```python
from build123d import *

# Parameters (mm, degrees)
SKETCH1_W                = 50
SKETCH1_H                = 50
BOSS_EXTRUDE1_DEPTH      = 50
CUT_EXTRUDE2_DEPTH       = 87.602540378
CUT_EXTRUDE3_DEPTH       = 40
CHAMFER1_SIZE            = 4
CHAMFER3_SIZE            = 1.5
BOSS_EXTRUDE2_DEPTH      = 7
BOSS_EXTRUDE2_DEPTH_BACK = 10
SKETCH5_W                = 1
SKETCH5_H                = 7
SKETCH6_W                = 1.8
SKETCH6_H                = 1.8
CUT_EXTRUDE4_DEPTH       = 7


with BuildPart() as part:
    # Sketch1 → Boss-Extrude1 (new body)
    with BuildSketch(Plane.XY):
        with Locations((25, 25)):
            Rectangle(SKETCH1_W, SKETCH1_H)
    extrude(amount=BOSS_EXTRUDE1_DEPTH)

    # Sketch3 → Cut-Extrude2 (cut, through all)
    with BuildSketch(Plane.XZ):
        Polygon((29.556349186, 39), (36, 45.443650814), (36, 54.556349186), (29.556349186, 61), (20.443650814, 61), (14, 54.556349186), (14, 45.443650814), (20.443650814, 39), align=None)
    extrude(amount=-CUT_EXTRUDE2_DEPTH, mode=Mode.SUBTRACT)

    # Sketch4 → Cut-Extrude3 (cut)
    with BuildSketch(Plane.XY.offset(50)):
        Polygon((33.69848481, 46), (16.30151519, 46), (4, 33.69848481), (4, 16.30151519), (16.30151519, 4), (33.69848481, 4), (46, 16.30151519), (46, 33.69848481), align=None)
    extrude(amount=-CUT_EXTRUDE3_DEPTH, mode=Mode.SUBTRACT)

    # Chamfer1
    chamfer1_edges = [part.edges().sort_by_distance(p)[0] for p in [
        (10.150757595, 10.150757595, 10),
        (10.150757595, 39.849242405, 10),
        (39.849242405, 39.849242405, 10),
        (39.849242405, 10.150757595, 10),
        (25, 4, 10),
        (25, 46, 10),
        (46, 25, 10),
        (4, 25, 10),
    ]]
    chamfer(chamfer1_edges, length=CHAMFER1_SIZE)

    # Chamfer3
    chamfer3_edges = [part.edges().sort_by_distance(p)[0] for p in [
        (50, 25, 50),
        (43, 50, 50),
        (43, 0, 50),
        (7, 50, 50),
        (36, 46.849242405, 50),
        (14, 3.150757595, 50),
        (14, 50, 47.721825407),
        (36, 50, 47.721825407),
        (36, 0, 47.721825407),
        (14, 0, 47.721825407),
        (17.221825407, 0, 42.221825407),
        (32.778174593, 0, 42.221825407),
        (17.221825407, 50, 42.221825407),
        (32.778174593, 50, 42.221825407),
        (0, 25, 50),
        (25, 50, 0),
        (50, 25, 0),
        (36, 3.150757595, 50),
        (14, 46.849242405, 50),
        (25, 0, 0),
        (9, 11.30151519, 50),
        (9, 38.69848481, 50),
        (4, 25, 50),
        (41, 38.69848481, 50),
        (0, 25, 0),
        (41, 11.30151519, 50),
        (46, 25, 50),
        (7, 0, 50),
        (0, 50, 25),
        (50, 50, 25),
        (50, 0, 25),
        (0, 0, 25),
    ]]
    chamfer(chamfer3_edges, length=CHAMFER3_SIZE)

    # Sketch5 → Boss-Extrude2 (add, two sides: drawn at the far end of the back side and taken through both)
    with BuildSketch(Plane.XY.offset(50).offset(-BOSS_EXTRUDE2_DEPTH_BACK)):
        with Locations((49.5, 25)):
            Rectangle(SKETCH5_W, SKETCH5_H)
    extrude(amount=BOSS_EXTRUDE2_DEPTH + BOSS_EXTRUDE2_DEPTH_BACK)

    # Sketch6 → Cut-Extrude4 (cut)
    with BuildSketch(Plane(origin=(50, 0, 0), x_dir=(0, 0, -1), z_dir=(1, 0, 0))):
        with Locations((-53.6, 25)):
            Rectangle(SKETCH6_W, SKETCH6_H)
    extrude(amount=-CUT_EXTRUDE4_DEPTH, mode=Mode.SUBTRACT)


solid = part.part
```
The model under review builds one solid part; all positions refer to its coordinate system, in mm. A direction names the side the tool comes from. Round coordinates to 2 decimals unless told otherwise and drop trailing zeros. Order: outer loops, then holes, each group sorted by start corner. A loop starts at its lowest first (then second) coordinate and runs counter-clockwise, first axis right, second up. Notation, with made-up numbers: (-9, -17.75) -> (16, -17.75) arc R24 ccw to (16, 16.25) -> close; hole circle Ø10 at (-7, -22). An arc over 180 degrees is marked (long way). One line per item, written item: value. Start each with the question number.
Q1. Take a section at D-D (y = 31). Write out the cut boundary in (x, z).
Q2. Take a section at A-A (y = 25). Write out the cut boundary in (x, z), and give its area (3 significant figures).
Q3. Take a section at C-C (x = 21.5). Write out the cut boundary in (y, z).
Q4. Mouldability with a two-part tool opening along X and no side actions: class faces 6 (the face through (10.2, 39.9, 31.5)), 7 (the face through (0.8, 0.7, 24.7)), 8 (the face through (42.9, 0.8, 49.3)) as released by +X, released by -X, zero draft, split by the parting line, or undercut.
Q5. Wall thickness on line 1 (X direction, y = 22, z = 17); line 2 (Z direction, x = 47, y = 4): over which ranges is each line inside the solid? List them lowest first.
Q6. Take a section at B-B (z = 26). Write out the cut boundary in (x, y), and give its area (3 significant figures).
Q7. Clearance check with flat-ended pins moving along their axes: pin 1 Ø0.5 at (x, z) = (49.5, 52) entering from -Y; pin 2 Ø0.5 at (x, z) = (49.5, 54) entering from +Y; pin 3 Ø5.5 at (x, y) = (45.5, 14) entering from +Z. State where each tip first meets the part, or that it passes through.
Q8. Machinability: for faces 1 (the face through (25, 46, 29)), 2 (the face through (6.9, 0.7, 49.2)), 3 (the face through (13, 1, 49)), 4 (the face through (36.7, 46.1, 49.2)), 5 (the face through (25, 25, 0)), which of the approach directions +Z, -Z, +X, -X, +Y, -Y give a long, thin tool a straight path to every point of the face, cutting with its end or side? Answer none if there is none.
Reported:
1. outline: (0, 1.5) -> (1.5, 0) -> (48.5, 0) -> (50, 1.5) -> (50, 48.5) -> (48.5, 50) -> (47.5, 50) -> (46, 48.5) -> (46, 14) -> (42, 10) -> (8, 10) -> (4, 14) -> (4, 48.5) -> (2.5, 50) -> (1.5, 50) -> (0, 48.5) -> close
2. outline: (0, 1.5) -> (1.5, 0) -> (48.5, 0) -> (50, 1.5) -> (50, 52.7) -> (49, 52.7) -> (49, 49.5) -> (48.5, 50) -> (47.5, 50) -> (46, 48.5) -> (46, 14) -> (42, 10) -> (8, 10) -> (4, 14) -> (4, 48.5) -> (2.5, 50) -> (1.5, 50) -> (0, 48.5) -> close; (49, 54.5) -> (50, 54.5) -> (50, 57) -> (49, 57) -> close
2. area: 835 mm2
3. outline: (0, 1.5) -> (1.5, 0) -> (48.5, 0) -> (50, 1.5) -> (50, 39) -> (46, 39) -> (46, 14) -> (42, 10) -> (8, 10) -> (4, 14) -> (4, 39) -> (0, 39) -> close
4. face 6: undercut
4. face 7: released by -X
4. face 8: zero draft
5. line 1: x = 0 to 4, 46 to 50
5. line 2: z = 0 to 50
6. outline: (0, 1.5) -> (1.5, 0) -> (48.5, 0) -> (50, 1.5) -> (50, 48.5) -> (48.5, 50) -> (1.5, 50) -> (0, 48.5) -> close; hole (4, 16.3) -> (16.3, 4) -> (33.7, 4) -> (46, 16.3) -> (46, 33.7) -> (33.7, 46) -> (16.3, 46) -> (4, 33.7) -> close
6. area: 1,030 mm2
7. pin 1: stops at y = 21.5
7. pin 2: stops at y = 28.5
7. pin 3: stops at z = 50
8. face 1: +Z
8. face 2: +Z, +X, -X, -Y
8. face 3: +Z, -Y
8. face 4: +Z, +Y, -Y
8. face 5: -Z, +X, -X, +Y, -Y
